Part model, mm, in its own coordinate system. A direction names the side the tool comes from. Round coordinates to 2 decimals unless told otherwise and drop trailing zeros. Write each loop counter-clockwise with the first axis right and the second up, starting at its lowest first coordinate (ties: lowest second). Pieces come first, ordered by that corner, then holes. Notation, with made-up numbers: M 70.25,22 L 109.25,22 A15 cw 109.25,32 Z; hole C 66,0.5 d7. An arc over 180 degrees is marked long. Use one line per item in the form item = value. Start each with the question number.
Item 1: Mould opens along Z. For faces 4 (the face through (0.251, -0.173, -1.546)), 5 (the face through (0, -2.778, -2)), 6 (the face through (0, 0, -5)) say: +Z half, -Z half, draft (parallel to the pull), parting line (faces both ways), or undercut.
Item 2: Flat gauge pins, fed straight in: pin 1 Ø1.5 at (x, z) = (1, -1.5) entering from -Y; pin 2 Ø4 at (y, z) = (3, 6.5) entering from -X; pin 3 Ø4 at (x, z) = (0.5, -2.5) entering from +Y. Where does each tip first touch, or does it go through?
Item 3: Probe L1, parallel to Z at x = 1, y = 0.5; L2, parallel to Z at x = -1.75, y = -2.5; L3, parallel to X at y = -0.5, z = -1. List the from-to ranges inside material, lowest first.
Item 4: Which spindle directions (+Z, -Z, +X, -X, +Y, -Y) get a long thin tool onto all of the face, cutting with end or side? Do faces 1 (the face through (0, 2.778, -2)), 2 (the face through (2.778, 0, -2)), 3 (the face through (-2.778, 0, -2)). Say none if no direction does.
Item 5: Cut at A-A, the plane z = 12.25. Give the cut face in (x, y), then the cut area to 3 significant figures.
from build123d import *

# Parameters (mm, degrees)
SKETCH1_W           = 5.55685425
SKETCH1_H           = 5.55685425
SKETCH3_W           = 5.55685425
SKETCH3_H           = 5.55685425
BOSS_EXTRUDE1_DEPTH = 5
BOSS_EXTRUDE2_DEPTH = 12
SKETCH5_R           = 1
CUT_EXTRUDE1_DEPTH  = 5


with BuildPart() as part:
    # Sketch1 → Loft1 section 0
    with BuildSketch(Plane.XY):
        Rectangle(SKETCH1_W, SKETCH1_H)
    # Sketch2 for Loft1 → Loft1 section 1
    with BuildSketch(Plane.XY.offset(2)):
        with BuildLine():
            # circular arc as an exact rational Bezier (weights 1, cos(half-angle), 1)
            Bezier((2.510229073, 2.510229073), (0, 5.020458147), (-2.510229073, 2.510229073), weights=[1, 0.707106781, 1])
            Bezier((-2.510229073, 2.510229073), (-5.020458147, 0), (-2.510229073, -2.510229073), weights=[1, 0.707106781, 1])
            Bezier((-2.510229073, -2.510229073), (0, -5.020458147), (2.510229073, -2.510229073), weights=[1, 0.707106781, 1])
            Bezier((2.510229073, -2.510229073), (5.020458147, 0), (2.510229073, 2.510229073), weights=[1, 0.707106781, 1])
        make_face()
    loft()

    # Sketch3 → Boss-Extrude1 (add)
    with BuildSketch(Plane(origin=(0, 0, 0), x_dir=(-1, 0, 0), z_dir=(0, 0, -1))):
        Rectangle(SKETCH3_W, SKETCH3_H)
    extrude(amount=BOSS_EXTRUDE1_DEPTH)

    # Sketch4 → Boss-Extrude2 (add)
    with BuildSketch(Plane.XY.offset(2)):
        with BuildLine():
            ThreePointArc((2.510229073, 2.510229073), (0, 3.55), (-2.510229073, 2.510229073))
            ThreePointArc((-2.510229073, 2.510229073), (-3.55, 0), (-2.510229073, -2.510229073))
            ThreePointArc((-2.510229073, -2.510229073), (0, -3.55), (2.510229073, -2.510229073))
            ThreePointArc((2.510229073, -2.510229073), (3.55, 0), (2.510229073, 2.510229073))
        make_face()
    extrude(amount=BOSS_EXTRUDE2_DEPTH)

    # Sketch5 → Cut-Extrude1 (cut, symmetric)
    with BuildSketch(Plane(origin=(0, 0, 0), x_dir=(0, 0, -1), z_dir=(0.7071067811865488, 0.7071067811865464, 0))):
        with Locations(Location((2.5, 0, 0), (0, 0, 180))):
            Circle(SKETCH5_R)
    extrude(amount=CUT_EXTRUDE1_DEPTH, both=True, mode=Mode.SUBTRACT)


solid = part.part
Model answer:
q1.face_4 = undercut
q1.face_5 = draft
q1.face_6 = -Z half
q2.pin_1 = -2.78
q2.pin_2 = -3.41
q2.pin_3 = 2.78
q3.L1 = -5 to -3.44, -1.56 to 14
q3.L2 = -5 to -3.35, -1.65 to 14
q3.L3 = -2.78 to 2.78
q4.face_1 = -Z, +X, -X, +Y
q4.face_2 = -Z, +X, +Y, -Y
q4.face_3 = -Z, -X, +Y, -Y
q5.outline = C 0,0 d7.1
q5.area = 39.6 mm²
